Check sheet for the modelled part. Datum: model origin and axes. Units: mm. Face numbers are marked on the shaded views. A direction names the side the tool comes from. Give positions to 0.01 mm unless a question says otherwise; leave off trailing zeros. Order: outer loops, then holes, each group sorted by start corner. A loop starts at its lowest first (then second) coordinate and runs counter-clockwise, first axis right, second up. Notation, with made-up numbers: (-27, -14) -> (-9, -14) arc R10 cw to (-9, 4) -> close; hole circle Ø11 at (71.5, 66.5). An arc over 180 degrees is marked (long way). One line per question, with ' | ' between items.
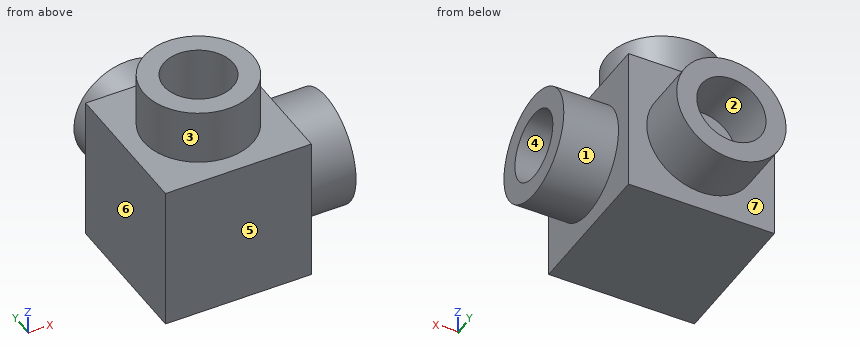
```python
from build123d import *

# Parameters (mm, degrees)
CROQUIS1_R              = 30
CROQUIS1_R_2            = 19
SALIENTE_EXTRUIR1_DEPTH = 30
CROQUIS2_W              = 80
CROQUIS2_H              = 80
SALIENTE_EXTRUIR2_DEPTH = 80
CROQUIS3_R              = 30
CROQUIS3_R_2            = 19
SALIENTE_EXTRUIR3_DEPTH = 30
CROQUIS4_R              = 30
CROQUIS4_R_2            = 19
SALIENTE_EXTRUIR4_DEPTH = 30


with BuildPart() as part:
    # Croquis1 → Saliente-Extruir1 (new body)
    with BuildSketch(Plane.XY):
        Circle(CROQUIS1_R)
        Circle(CROQUIS1_R_2, mode=Mode.SUBTRACT)
    extrude(amount=SALIENTE_EXTRUIR1_DEPTH)

    # Croquis2 → Saliente-Extruir2 (add)
    with BuildSketch(Plane.XY):
        Rectangle(CROQUIS2_W, CROQUIS2_H)
    extrude(amount=-SALIENTE_EXTRUIR2_DEPTH)

    # Croquis3 → Saliente-Extruir3 (add)
    with BuildSketch(Plane(origin=(40, 0, 0), x_dir=(0, 0, -1), z_dir=(1, 0, 0))):
        with Locations((40, 0)):
            Circle(CROQUIS3_R)
        with Locations(Location((40, 0, 0), (0, 0, 90))):
            Circle(CROQUIS3_R_2, mode=Mode.SUBTRACT)
    extrude(amount=SALIENTE_EXTRUIR3_DEPTH)

    # Croquis4 → Saliente-Extruir4 (add)
    with BuildSketch(Plane(origin=(0, 40, 0), x_dir=(1, 0, 0), z_dir=(0, 1, 0))):
        with Locations(Location((0, 40, 0), (0, 0, 270))):
            Circle(CROQUIS4_R)
        with Locations(Location((0, 40, 0), (0, 0, 270))):
            Circle(CROQUIS4_R_2, mode=Mode.SUBTRACT)
    extrude(amount=SALIENTE_EXTRUIR4_DEPTH)


solid = part.part
```
Q1. Access from +Z, -Z, +X, -X, +Y, -Y to the whole of each face (thin tool, end or side, straight path). Record for the marked faces 1, 2 and 3.
Result sheet:
face 1: +X | face 2: +Y | face 3: +Z
Q2. Section check C-C (z = 18.5). Enter the section's corners in (x, y).
Result sheet:
outline: circle Ø60 at (0, 0); hole circle Ø38 at (0, 0)
Q3. Mould release check, pull along Y, two halves, no side actions. Record for the marked faces 4, 5, 6 and 7: pulls with the +Y half, pulls with the -Y half, needs draft (parallel to the pull), parting line crosses it, or undercut.
Result sheet:
face 4: undercut | face 5: pulls with the -Y half | face 6: needs draft | face 7: pulls with the +Y half
Q4. Section check D-D (z = -73). Enter the section's corners in (x, y).
Result sheet:
outline: (-40, -40) -> (40, -40) -> (40, 40) -> (-40, 40) -> close
Q5. Thickness scan on line 1 (X direction, y = 56, z = -40); line 2 (X direction, y = 18.5, z = -69). Record the ranges inside material, lowest first.
Result sheet:
line 1: x = -30 to -19, 19 to 30 | line 2: x = -40 to 40
Q6. Section check A-A (x = 0). Enter the section's corners in (y, z), and give its area (3 significant figures).
Result sheet:
outline: (-40, -80) -> (40, -80) -> (40, -70) -> (70, -70) -> (70, -59) -> (40, -59) -> (40, -21) -> (70, -21) -> (70, -10) -> (40, -10) -> (40, 0) -> (30, 0) -> (30, 30) -> (19, 30) -> (19, 0) -> (-19, 0) -> (-19, 30) -> (-30, 30) -> (-30, 0) -> (-40, 0) -> close | area: 7,720 mm2
Q7. Depth check by flat-ended pin: pin 1 Ø3 at (x, z) = (37, -19) entering from +Y; pin 2 Ø19 at (x, y) = (-7, 3.5) entering from +Z; pin 3 Ø8 at (y, z) = (56, -18) entering from +X. Enter the tip coordinate at first touch or a pass-through.
Result sheet:
pin 1: stops at y = 40 | pin 2: stops at z = 0 | pin 3: stops at x = 24
